Can you work these out from the drawing? Everything is in mm from the part's minimum corner. Round coordinates to 2 decimals unless told otherwise and drop trailing zeros. Order: outer loops, then holes, each group sorted by start corner. A loop starts at its lowest first (then second) coordinate and runs counter-clockwise, first axis right, second up. Notation, with made-up numbers: (47.25, 82.25) -> (82.25, 82.25) arc R35 ccw to (82.25, 120.25) -> close; hole circle Ø5 at (26, 48.25). An arc over 180 degrees is marked (long way). One line per item, written item: value.
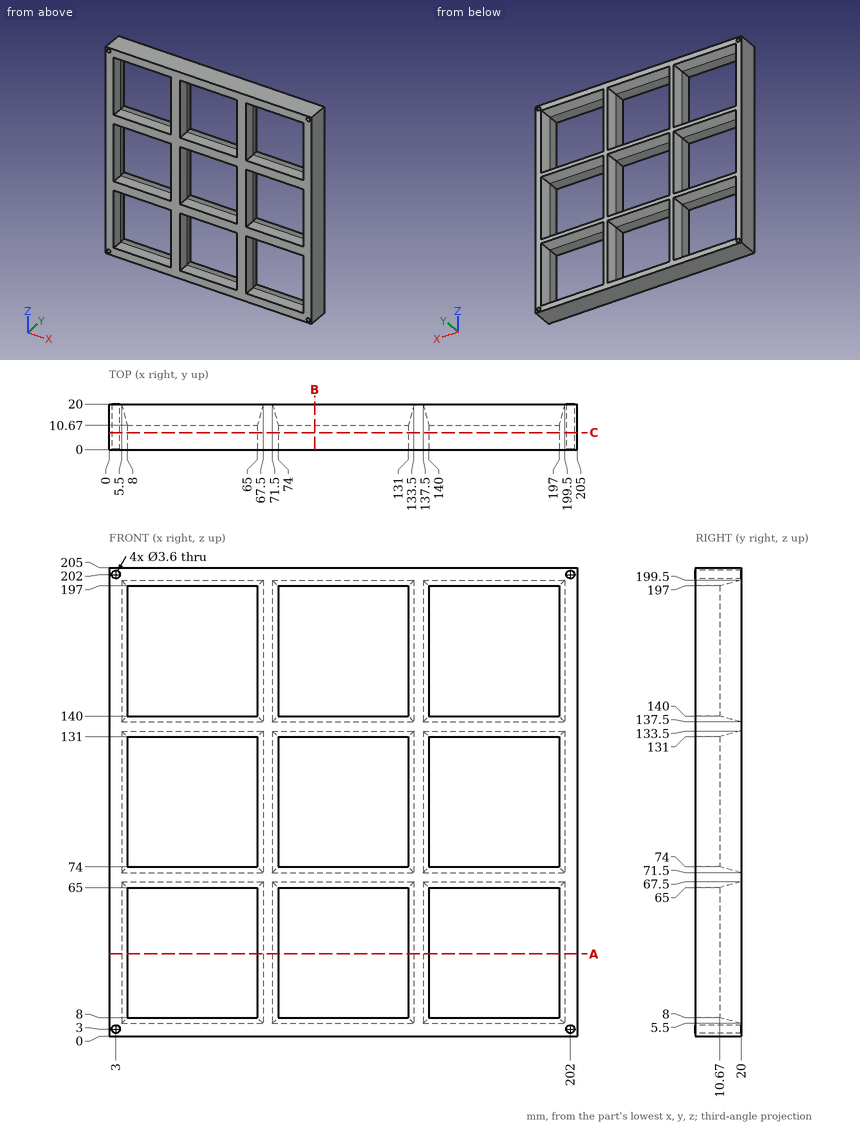
Q1. Please list where these lines run through material, in increasing order: line 1 along X through (y, z) = (7.75, 56.5); line 2 along X through (y, z) = (10.5, 202).
Answers below:
line 1: 0 to 8, 65 to 74, 131 to 140, 197 to 205
line 2: 0 to 1.2, 4.8 to 200.2, 203.8 to 205
Q2. I want a section at B-B on x = 90. List the corners of the cut face in (y, z) for me.
Answers below:
outline: (0, 0) -> (20, 0) -> (20, 5.5) -> (10.67, 8) -> (0, 8) -> close; (0, 65) -> (10.67, 65) -> (20, 67.5) -> (20, 71.5) -> (10.67, 74) -> (0, 74) -> close; (0, 131) -> (10.67, 131) -> (20, 133.5) -> (20, 137.5) -> (10.67, 140) -> (0, 140) -> close; (0, 197) -> (10.67, 197) -> (20, 199.5) -> (20, 205) -> (0, 205) -> close
Q3. I want a section at C-C on y = 7.5. Give the number of separate pieces and of enclosed holes in the cut face, plus the area to 3 significant figures.
Answers below:
separate pieces: 1
enclosed holes: 13
area: 12,700 mm^2
Q4. I want a section at A-A on z = 36. List the corners of the cut face in (x, y) for me, plus the area to 3 significant figures.
Answers below:
outline: (0, 0) -> (8, 0) -> (8, 10.67) -> (5.5, 20) -> (0, 20) -> close; (65, 0) -> (74, 0) -> (74, 10.67) -> (71.5, 20) -> (67.5, 20) -> (65, 10.67) -> close; (131, 0) -> (140, 0) -> (140, 10.67) -> (137.5, 20) -> (133.5, 20) -> (131, 10.67) -> close; (197, 0) -> (205, 0) -> (205, 20) -> (199.5, 20) -> (197, 10.67) -> close
area: 610 mm^2
